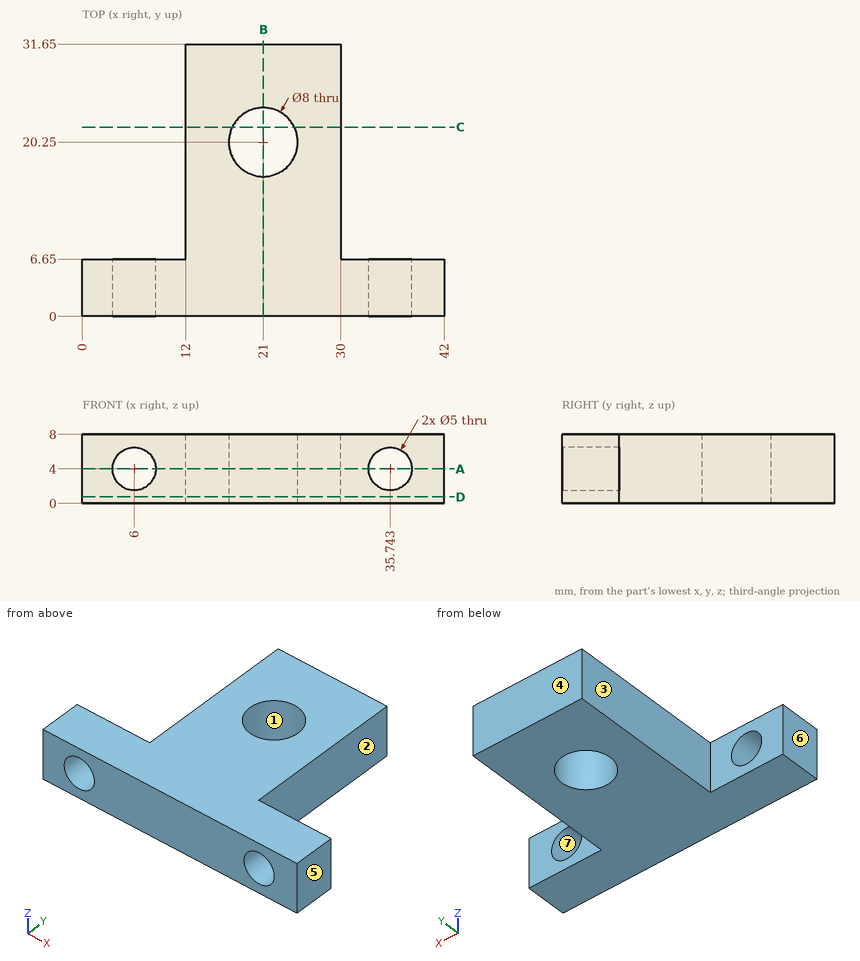
Answer from the drawing. Dimensions are ordinates in mm from the lowest x, y and z of the part. A direction names the side the tool comes from. Give positions to 0.01 mm unless a question says otherwise; leave off trailing zeros. Order: outer loops, then holes, each group sorted by start corner. A loop starts at its lowest first (then second) coordinate and runs counter-clockwise, first axis right, second up.
(1) Find section C-C (y = 22). Give the vertices of the cut face in (x, z).
(2) Straight lines are drawn through the part: L1, parallel to X at y = 2.25, z = 4; L2, parallel to Y at x = 21, z = 3.75; L3, parallel to X at y = 27.5, z = 3. For each, find the intervals that lie inside material, in ascending order.
(3) Find section D-D (z = 0.75). Give the vertices of the cut face in (x, y), plus the area to 3 significant figures.
(4) Given pin 1 (4 mm diameter, centred on y = 25, z = 3, fed in from +X); pin 2 (2.5 mm diameter, centred on y = 19.5, z = 4.5, fed in from -X), each flat-ended and moving along its own axis, determine where each tip first touches the part or whether it passes through.
(5) Find section B-B (x = 21). Give the vertices of the cut face in (y, z), plus the area to 3 significant figures.
(6) For a pull along X with two mould halves and no side action, classify the marked faces 4, 5, 6 and 7 as released by +X, released by -X, zero draft, split by the parting line, or undercut.
(7) For the marked faces 1, 2 and 3, determine the directions among +Z, -Z, +X, -X, +Y, -Y from which every point of the face is accessible in a straight line to the end or side of a thin tool.
(8) Find section A-A (z = 4). Give the vertices of the cut face in (x, y).
Result sheet:
1. outline: (12, 0) - (17.4, 0) - (17.4, 8) - (12, 8) - close; (24.6, 0) - (30, 0) - (30, 8) - (24.6, 8) - close
2. L1: x = 0 to 3.5, 8.5 to 33.24, 38.24 to 42
2. L2: y = 0 to 16.25, 24.25 to 31.65
2. L3: x = 12 to 30
3. outline: (0, 0) - (42, 0) - (42, 6.65) - (30, 6.65) - (30, 31.65) - (12, 31.65) - (12, 6.65) - (0, 6.65) - close; hole circle Ø8 at (21, 20.25)
3. area: 679 mm2
4. pin 1: stops at x = 30
4. pin 2: stops at x = 12
5. outline: (0, 0) - (16.25, 0) - (16.25, 8) - (0, 8) - close; (24.25, 0) - (31.65, 0) - (31.65, 8) - (24.25, 8) - close
5. area: 189 mm2
6. face 4: zero draft
6. face 5: released by +X
6. face 6: released by -X
6. face 7: undercut
7. face 1: +Z, -Z
7. face 2: +Z, -Z, +X, +Y
7. face 3: +Z, -Z, -X, +Y
8. outline: (0, 0) - (3.5, 0) - (3.5, 6.65) - (0, 6.65) - close; (8.5, 0) - (33.24, 0) - (33.24, 6.65) - (30, 6.65) - (30, 31.65) - (12, 31.65) - (12, 6.65) - (8.5, 6.65) - close; (38.24, 0) - (42, 0) - (42, 6.65) - (38.24, 6.65) - close; hole circle Ø8 at (21, 20.25)
